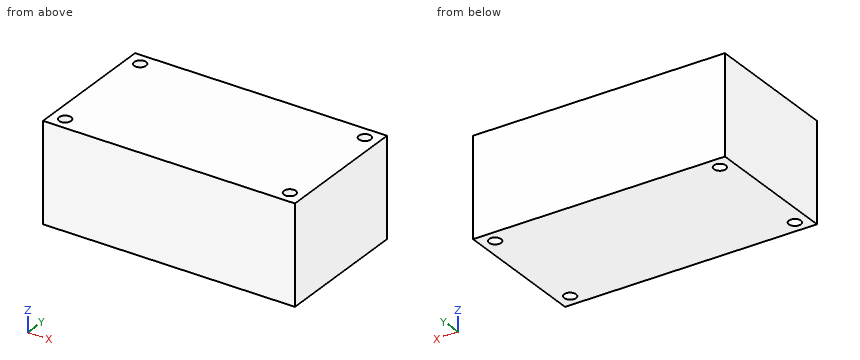
```python
from build123d import *

# Parameters (mm, degrees)
SKETCH_1_W      = 74
SKETCH_1_H      = 40.5
SKETCH_1_R      = 1.75
EXTRUDE_1_DEPTH = 29


with BuildPart() as part:
    # 草圖1 → 伸長1 (new body)
    with BuildSketch(Plane.XY):
        Rectangle(SKETCH_1_W, SKETCH_1_H)
        with Locations(Location((-33, 16.5, 0), (0, 0, 180))):
            Circle(SKETCH_1_R, mode=Mode.SUBTRACT)
        with Locations(Location((-33, -16.5, 0), (0, 0, 180))):
            Circle(SKETCH_1_R, mode=Mode.SUBTRACT)
        with Locations(Location((33, -16.5, 0), (0, 0, 180))):
            Circle(SKETCH_1_R, mode=Mode.SUBTRACT)
        with Locations(Location((33, 16.5, 0), (0, 0, 180))):
            Circle(SKETCH_1_R, mode=Mode.SUBTRACT)
    extrude(amount=EXTRUDE_1_DEPTH)


solid = part.part
```
Part model, mm, in its own coordinate system. Coordinates: 2 decimals unless noted, no trailing zeros. Write each loop counter-clockwise with the first axis right and the second up, starting at its lowest first coordinate (ties: lowest second). Pieces come first, ordered by that corner, then holes.
Item 1: Pin check, flat tip, straight feed: pin 1 (4 mm diameter, centred on x = -33, y = -16.5, fed in from +Z). Stop position of the tip, or through.
Item 2: Slice it at B-B (y = -16.5). Write the cut outline in (x, z).
Item 3: Probe line 1 (X direction, y = -16.5, z = 20); line 2 (Y direction, x = 33, z = 14). List the from-to ranges inside material, lowest first.
Item 4: Slice it at A-A (x = -33). Write the cut outline in (y, z).
Results found:
1. pin 1: stops at z = 29
2. outline: (-37, 0) - (-34.75, 0) - (-34.75, 29) - (-37, 29) - close; (-31.25, 0) - (31.25, 0) - (31.25, 29) - (-31.25, 29) - close; (34.75, 0) - (37, 0) - (37, 29) - (34.75, 29) - close
3. line 1: x = -37 to -34.75, -31.25 to 31.25, 34.75 to 37
3. line 2: y = -20.25 to -18.25, -14.75 to 14.75, 18.25 to 20.25
4. outline: (-20.25, 0) - (-18.25, 0) - (-18.25, 29) - (-20.25, 29) - close; (-14.75, 0) - (14.75, 0) - (14.75, 29) - (-14.75, 29) - close; (18.25, 0) - (20.25, 0) - (20.25, 29) - (18.25, 29) - close
